Can you work these out from the model? Positions are in its coordinate system, mm. A direction names the side the tool comes from. Give positions to 0.01 mm unless a question says otherwise; leave off trailing zeros. Order: outer loops, then holes, each group sorted by start corner. A loop starts at its lowest first (then second) coordinate and runs counter-clockwise, first axis right, second up. Notation, with made-up numbers: M 79,78 L 83,78 A26 ccw 83,114 Z; hole C 26,-15 d11. An arc over 180 degrees is marked long. Answer as a JSON object with one key per item and string values.
Autodesk Inventor part; units mm, degrees
ref_plane "YZ Plane" through (0, 0, 0) normal (1, 0, 0) x (0, 1, 0)
ref_plane "XZ Plane" through (0, 0, 0) normal (0, 1, 0) x (-1, 0, 0)
ref_plane "XY Plane" through (0, 0, 0) normal (0, 0, 1) x (1, 0, 0)
sketch "Sketch1" plane through (0, 0, 0) normal (1, 0, 0) x (0, 1, 0)
  line L0 (0, -0.4446) -> (0, -24.9554)
  line L1 (-0.4178, -25.5521) -> (-4.3558, -26.9854)
  line L2 (-0.4178, 0.1521) -> (-4.3558, 1.5854)
  line L3 (-5.0594, 1.3969) -> (-6.4063, -0.2083)
  line L4 (-4.8497, -23.8856) -> (-4.8389, -24.1212)
  line L5 (-3.9874, -24.6889) -> (-2.4498, -24.1293)
  line L6 (-2.032, -23.5325) -> (-2.032, -1.8675)
  line L7 (-2.4498, -1.2707) -> (-3.7138, -0.8107)
  line L8 (-4.4174, -0.9992) -> (-4.8497, -1.5144)
  line L9 (-6.4063, -0.2083) -> (-4.8497, -1.5144)
  arc A0 (0, -0.4446) -> (-0.4178, 0.1521) centre (-0.635, -0.4446) ccw
  arc A1 (-2.032, -1.8675) -> (-2.4498, -1.2707) centre (-2.667, -1.8675) ccw
  arc A2 (-4.3558, 1.5854) -> (-5.0594, 1.3969) centre (-4.573, 0.9887) ccw
  arc A3 (-3.7138, -0.8107) -> (-4.4174, -0.9992) centre (-3.931, -1.4074) ccw
  arc A4 (-2.4498, -24.1293) -> (-2.032, -23.5325) centre (-2.667, -23.5325) ccw
  arc A5 (-0.4178, -25.5521) -> (0, -24.9554) centre (-0.635, -24.9554) ccw
  arc A6 (-4.8389, -24.1212) -> (-3.9874, -24.6889) centre (-4.2046, -24.0922) ccw
  line L10 (-4.8497, -23.8856) -> (-4.8497, -1.5144)
  line L11 (-9.6994, -0.4446) -> (-9.6994, -24.9554)
  line L12 (-9.2816, -25.5521) -> (-5.3436, -26.9854)
  line L13 (-9.2816, 0.1521) -> (-5.3436, 1.5854)
  line L14 (-4.64, 1.3969) -> (-3.2931, -0.2083)
  line L15 (-5.712, -24.6889) -> (-7.2496, -24.1293)
  line L16 (-7.6674, -23.5325) -> (-7.6674, -1.8675)
  line L17 (-7.2496, -1.2707) -> (-5.9856, -0.8107)
  line L18 (-5.282, -0.9992) -> (-4.8497, -1.5144)
  line L19 (-3.2931, -0.2083) -> (-4.8497, -1.5144)
  arc A7 (-9.2816, 0.1521) -> (-9.6994, -0.4446) centre (-9.0644, -0.4446) ccw
  arc A8 (-7.2496, -1.2707) -> (-7.6674, -1.8675) centre (-7.0324, -1.8675) ccw
  arc A9 (-4.64, 1.3969) -> (-5.3436, 1.5854) centre (-5.1264, 0.9887) ccw
  arc A10 (-5.282, -0.9992) -> (-5.9856, -0.8107) centre (-5.7685, -1.4074) ccw
  arc A11 (-7.6674, -23.5325) -> (-7.2496, -24.1293) centre (-7.0324, -23.5325) ccw
  arc A12 (-9.6994, -24.9554) -> (-9.2816, -25.5521) centre (-9.0644, -24.9554) ccw
  arc A13 (-5.712, -24.6889) -> (-4.8605, -24.1212) centre (-5.4948, -24.0922) ccw
  line L20 (-5.3436, -26.9854) -> (-4.3558, -26.9854)
  line L21 (0, -12.7) -> (-9.6994, -12.7)
  line L22 (-5.0594, -26.7969) -> (-6.4063, -25.1917)
  line L23 (-4.8389, -24.1212) -> (-4.8497, -23.8856)
  line L24 (-6.4063, -25.1917) -> (-4.8497, -23.8856)
  arc A14 (-5.0594, -26.7969) -> (-4.3558, -26.9854) centre (-4.573, -26.3887) ccw
  arc A15 (-5.3436, -26.9854) -> (-4.64, -26.7969) centre (-5.1264, -26.3887) ccw
  line L25 (-4.64, -26.7969) -> (-3.2931, -25.1917)
  line L26 (-4.8605, -24.1212) -> (-4.8497, -23.8856)
  line L27 (-3.2931, -25.1917) -> (-4.8497, -23.8856)
  point P0 (0, 0)
  point P1 (0, -25.4)
  point P2 (-4.7736, -27.1375)
  point P3 (-4.7736, 1.7375)
  point P4 (-4.7995, -24.9845)
  point P5 (-2.032, -23.9772)
  point P6 (-2.032, -1.4228)
  point P7 (-4.1316, -0.6586)
  dimension "d0" = 25.4
  dimension "d4" = 5.08
  dimension "d5" = 110
  dimension "d8" = 5.08
  dimension "d10" = 110
  dimension "d11" = 2.54
  dimension "d12" = 110
  dimension "d13" = 2.032
  dimension "d16" = 0.635
  dimension "d18" = 2.032
extrude "Extrusion1" add sketch "Sketch1" along normal blind 878.84 contours L0 L21 L6 A1 L7 A3 L19 L14 A9 A2 L2 A0 | L0 A5 L1 L20 A14 A15 L25 L27 L5 A4 L6 L21 | A9 L14 L19 A3 L8 L18 A10 L9 L3 A2 | A2 L3 L9 A10 L17 A8 L16 L21 L11 A7 L13 A9 | A14 L20 | L27 L5 A6 L4 | L26 A13 L15 L24 | L4 A6 L5 L27 L25 A15 A14 L22 L24 L15 A13 L26 | L9 A10 L18 | L8 A3 L19 | L16 A11 L15 L24 L22 A14 A15 L20 L12 A12 L11 L21 | A15 L20
properties part number "the smaller outside slider part"
1) I want a section at A-A on z = -18.75. Write out the boundary of the cut face in (x, y), and give its area (3 significant figures).
Results found:
{"outline": "M 0,-9.7 L 878.84,-9.7 L 878.84,-7.67 L 0,-7.67 Z; M 0,-2.03 L 878.84,-2.03 L 878.84,0 L 0,0 Z", "area": "3,570 mm²"}
2) I'm going to push a flat-ended pin straight in: pin 1 Ø2 at (x, y) = (573.5, -2) entering from +Z. Where does the tip first touch, or does it pass through?
Results found:
{"pin 1": "stops at z = 1.09"}
3) Thinking about a two-plate mould opening in Z: for faces 1 (the face through (433, -7.667, -13)), 2 (the face through (433, 0, -13)), which applies, pulls with the +Z half, pulls with the -Z half, needs draft (parallel to the pull), parting line crosses it, or undercut?
Results found:
{"face 1": "undercut", "face 2": "needs draft"}
4) I need wall thicknesses on L1, parallel to Y at x = 484.5, z = -2; L2, parallel to Z at x = 244.5, y = -5.75; L3, parallel to Z at x = 269.5, y = -4. Which ranges of each line are inside material? Lowest first, please.
Results found:
{"L1": "y = -9.7 to -7.67, -2.03 to 0", "L2": "z = -26.84 to -24.64, -0.77 to 1.44", "L3": "z = -26.86 to -24.6, -0.8 to 1.46"}
5) For faces 3 (the face through (433, -9.699, -13)), 4 (the face through (433, -2.032, -13)), which set-ups out of +Z, -Z, +X, -X, +Y, -Y let a thin tool reach every point of the face, with its end or its side?
Results found:
{"face 3": "+Z, -Z, +X, -X, -Y", "face 4": "+X, -X"}
